Part model, mm, in its own coordinate system. Round coordinates to 2 decimals unless told otherwise and drop trailing zeros. Loops run counter-clockwise (first coordinate to the right, second up) from the corner with the lowest first, then second, coordinate; pieces in that order, holes last.
1) Probe line 1 (Z direction, x = 0, y = -12.75); line 2 (X direction, y = -14.75, z = 2.5); line 3 (X direction, y = -16, z = -3). List the from-to ranges inside material, lowest first.
2) Band-saw the part on B-B, the plane y = -14.25. Write the cut outline in (x, z), then the cut area to 3 significant figures.
3) Band-saw the part on C-C, the plane y = -4. Write the cut outline in (x, z).
4) Band-saw the part on A-A, the plane x = 0. Write the cut outline in (y, z), then the cut area to 3 significant figures.
5) Band-saw the part on D-D, the plane y = -22.75. Write the cut outline in (x, z), then the cut area to 3 significant figures.
6) Drop flat-ended pins along their axis: P1, Ø6, axis at y = -19.5, z = 3, coming from the -X side; P2, Ø3, axis at x = 16.5, y = -21.5, coming from the -Z side; P3, Ø12, axis at y = -16, z = 22.5, coming from the +X side. Give the stop position or say it passes through.
from build123d import *

# Parameters (mm, degrees)
F0_W     = 60
F0_H     = 60
F1_DEPTH = 25
F2_R     = 44.839228
F3_R     = 20.655466
F5_R     = 15.261673
F6_DEPTH = 30


with BuildPart() as f1:
    # F0 (on Front) → F1 (new body)
    with BuildSketch(Plane.XZ):
        Rectangle(F0_W, F0_H)
    extrude(amount=F1_DEPTH)

    # F2 (on Front) → F4 section 0
    with BuildSketch(Plane.XZ):
        Circle(F2_R)
    # F3 (on face) → F4 section 1
    with BuildSketch(Plane.XZ.offset(25)):
        Circle(F3_R)
    loft(mode=Mode.INTERSECT)

    # F5 (on face) → F6 (cut)
    with BuildSketch(Plane.XZ.offset(25)):
        Circle(F5_R)
    extrude(amount=-F6_DEPTH, mode=Mode.SUBTRACT)


solid = f1.part
Reported:
1. line 1: z = -30 to -15.26, 15.26 to 30
1. line 2: x = -30 to -15.06, 15.06 to 30
1. line 3: x = -29.21 to -14.96, 14.96 to 29.21
2. outline: (-30, -8.02) arc R31.05 ccw to (-8.02, -30) - (8.02, -30) arc R31.05 ccw to (30, -8.02) - (30, 8.02) arc R31.05 ccw to (8.02, 30) - (-8.02, 30) arc R31.05 ccw to (-30, 8.02) - close; hole circle Ø30.52 at (0, 0)
2. area: 2,250 mm2
3. outline: (-30, -27.9) arc R40.97 ccw to (-27.9, -30) - (27.9, -30) arc R40.97 ccw to (30, -27.9) - (30, 27.9) arc R40.97 ccw to (27.9, 30) - (-27.9, 30) arc R40.97 ccw to (-30, 27.9) - close; hole circle Ø30.52 at (0, 0)
4. outline: (-25, -20.66) - (-15.34, -30) - (0, -30) - (0, -15.26) - (-25, -15.26) - close; (-25, 15.26) - (0, 15.26) - (0, 30) - (-15.34, 30) - (-25, 20.66) - close
4. area: 647 mm2
5. outline: circle Ø45.66 at (0, 0); hole circle Ø30.52 at (0, 0)
5. area: 906 mm2
6. P1: stops at x = -28.74
6. P2: stops at z = -19.8
6. P3: stops at x = 28.32
